from build123d import *

# Parameters (mm, degrees)
SKETCH1_W               = 94
SKETCH1_H               = 57
BOSS_EXTRUDE1_DEPTH     = 10
BOSS_EXTRUDE2_DEPTH     = 30
SKETCH3_W               = 1.5
SKETCH3_H               = 1.4
SKETCH3_W_2             = 1
SKETCH3_H_2             = 1
BOSS_EXTRUDE3_DEPTH     = 92
SKETCH3_3_W             = 1
SKETCH3_3_H             = 1
BOSS_EXTRUDE4_DEPTH     = 10
SKETCH4_W               = 46
SKETCH4_H               = 11
CUT_EXTRUDE1_DEPTH      = 10
SKETCH5_W               = 2
SKETCH5_H               = 2
CUT_EXTRUDE2_DEPTH      = 2
BOSS_EXTRUDE5_DEPTH     = 2
FILLET1_SIZE            = 1.5
BOSS_EXTRUDE6_DEPTH     = 1
SKETCH9_W               = 10
SKETCH9_H               = 2
BOSS_EXTRUDE7_DEPTH     = 2
CUT_EXTRUDE3_DEPTH      = 79.407264077
CUT_EXTRUDE3_DEPTH_BACK = 79.407264077
SKETCH10_W              = 52
SKETCH10_H              = 34
SKETCH11_W              = 92
SKETCH11_H              = 50
CUT_EXTRUDE4_DEPTH      = 2.2


with BuildPart() as part:
    # Sketch1 → Boss-Extrude1 (new body)
    with BuildSketch(Plane(origin=(0, 0, 0), x_dir=(1, 0, 0), z_dir=(0, 1, 0))):
        with Locations((16.701972288, 4.145945946)):
            Rectangle(SKETCH1_W, SKETCH1_H)
    extrude(amount=BOSS_EXTRUDE1_DEPTH)

    # Sketch2 → Boss-Extrude2 (add)
    with BuildSketch(Plane(origin=(0, 10, 0), x_dir=(1, 0, 0), z_dir=(0, 1, 0))):
        Polygon((-30.298027712, 32.645945946), (63.701972288, 32.645945946), (63.701972288, -24.354054054), (-30.298027712, -24.354054054), (-30.298027712, -22.354054054), (61.701972288, -22.354054054), (61.701972288, 30.645945946), (-30.298027712, 30.645945946), align=None)
    extrude(amount=BOSS_EXTRUDE2_DEPTH)

    # Sketch3 → Boss-Extrude3 (add)
    with BuildSketch(Plane.ZY.offset(30.298027712)):
        with Locations((-29.895945946, 10.7)):
            Rectangle(SKETCH3_W, SKETCH3_H)
        with Locations((21.604054054, 10.7)):
            Rectangle(SKETCH3_W, SKETCH3_H)
        with Locations((21.854054054, 14)):
            Rectangle(SKETCH3_W_2, SKETCH3_H_2)
    extrude(amount=-BOSS_EXTRUDE3_DEPTH)

    # Sketch3<3> → Boss-Extrude4 (add)
    with BuildSketch(Plane.ZY.offset(30.298027712)):
        with Locations((-30.145945946, 14)):
            Rectangle(SKETCH3_3_W, SKETCH3_3_H)
    extrude(amount=-BOSS_EXTRUDE4_DEPTH)

    # Sketch4 → Cut-Extrude1 (cut)
    with BuildSketch(Plane(origin=(0, 0, -32.645945946), x_dir=(-1, 0, 0), z_dir=(0, 0, -1))):
        with Locations((-33.701972288, 29)):
            Rectangle(SKETCH4_W, SKETCH4_H)
    extrude(amount=-CUT_EXTRUDE1_DEPTH, mode=Mode.SUBTRACT)

    # Sketch5 → Cut-Extrude2 (cut)
    with BuildSketch(Plane(origin=(63.701972288, 0, 0), x_dir=(0, 0, -1), z_dir=(1, 0, 0))):
        Polygon((-2.854054054, 30), (11.145945946, 30), (13.145945946, 28), (13.145945946, 14), (-4.854054054, 14), (-4.854054054, 28), align=None)
        with Locations((-7.854054054, 21)):
            Rectangle(SKETCH5_W, SKETCH5_H)
        with Locations((16.145945946, 21)):
            Rectangle(SKETCH5_W, SKETCH5_H)
    extrude(amount=-CUT_EXTRUDE2_DEPTH, mode=Mode.SUBTRACT)

    # Sketch7 → Boss-Extrude5 (add)
    with BuildSketch(Plane(origin=(0, 33, 0), x_dir=(1, 0, 0), z_dir=(0, 1, 0))):
        Polygon((10.701972288, -22.354054054), (61.701972288, -22.354054054), (61.701972288, -20.354054054), (61.701972288, 15.645945946), (59.701972288, 15.645945946), (59.701972288, -20.354054054), (10.701972288, -20.354054054), align=None)
    extrude(amount=-BOSS_EXTRUDE5_DEPTH)

    # Fillet1
    # a fillet whose section is not a circle: 1.5 mm, written as the material it takes off along each edge
    with BuildSketch(Plane(origin=(59.701972288, 31, -19.395945946), x_dir=(1, 0, 0), z_dir=(0, 0, 1))) as fillet1_piece_1:
        with BuildLine():
            Bezier((FILLET1_SIZE, 0), (0, 0), (0, FILLET1_SIZE), weights=[1, 0.353553391, 1])
            Line((0, FILLET1_SIZE), (0, 0))
            Line((0, 0), (FILLET1_SIZE, 0))
        make_face()
    extrude(amount=39.75, mode=Mode.SUBTRACT)
    with BuildSketch(Plane(origin=(59.701972288, 31, 20.354054054), x_dir=(0, 0, 1), z_dir=(-1, 0, 0))) as fillet1_piece_2:
        with BuildLine():
            Bezier((FILLET1_SIZE, 0), (0, 0), (0, FILLET1_SIZE), weights=[1, 0.353553391, 1])
            Line((0, FILLET1_SIZE), (0, 0))
            Line((0, 0), (FILLET1_SIZE, 0))
        make_face()
    extrude(amount=52.75, mode=Mode.SUBTRACT)
    with BuildSketch(Plane(origin=(59.701972288, 31, -19.395945946), x_dir=(1, 0, 0), z_dir=(0, 0, 1))) as fillet1_piece_3a_section:
        with BuildLine():
            Bezier((FILLET1_SIZE, 0), (0, 0), (0, FILLET1_SIZE), weights=[1, 0.353553391, 1])
            Line((0, FILLET1_SIZE), (0, 0))
            Line((0, 0), (FILLET1_SIZE, 0))
        make_face()
    fillet1_piece_3a = extrude(amount=43.5, mode=Mode.PRIVATE)
    fillet1_piece_3a = split(fillet1_piece_3a, bisect_by=Plane(origin=(59.701972288, 31, 22.354054054), z_dir=(0, 0, -1)), keep=Keep.TOP, mode=Mode.PRIVATE)
    fillet1_piece_3a = split(fillet1_piece_3a, bisect_by=Plane(origin=(59.701972288, 31, 20.354054054), z_dir=(0, 0, 1)), keep=Keep.TOP, mode=Mode.PRIVATE)
    with BuildSketch(Plane(origin=(63.451972288, 31, 20.354054054), x_dir=(0, 0, 1), z_dir=(-1, 0, 0))) as fillet1_piece_3b_section:
        with BuildLine():
            Bezier((FILLET1_SIZE, 0), (0, 0), (0, FILLET1_SIZE), weights=[1, 0.353553391, 1])
            Line((0, FILLET1_SIZE), (0, 0))
            Line((0, 0), (FILLET1_SIZE, 0))
        make_face()
    fillet1_piece_3b = extrude(amount=56.5, mode=Mode.PRIVATE)
    fillet1_piece_3b = split(fillet1_piece_3b, bisect_by=Plane(origin=(61.701972288, 31, 20.354054054), z_dir=(-1, 0, 0)), keep=Keep.TOP, mode=Mode.PRIVATE)
    fillet1_piece_3b = split(fillet1_piece_3b, bisect_by=Plane(origin=(59.701972288, 31, 20.354054054), z_dir=(1, 0, 0)), keep=Keep.TOP, mode=Mode.PRIVATE)
    fillet1_piece_3 = fillet1_piece_3a & fillet1_piece_3b
    add(fillet1_piece_3, mode=Mode.SUBTRACT)

    # Sketch8 → Boss-Extrude6 (add)
    with BuildSketch(Plane(origin=(0, 34.8, 0), x_dir=(1, 0, 0), z_dir=(0, 1, 0))):
        Polygon((10.701972288, -20.354054054), (59.701972288, -20.354054054), (59.701972288, 15.645945946), (61.701972288, 15.645945946), (61.701972288, -22.354054054), (10.701972288, -22.354054054), align=None)
    extrude(amount=BOSS_EXTRUDE6_DEPTH)

    # Sketch9 → Boss-Extrude7 (add)
    with BuildSketch(Plane(origin=(0, 40, 0), x_dir=(1, 0, 0), z_dir=(0, 1, 0))):
        with Locations((-25.298027712, 31.645945946)):
            Rectangle(SKETCH9_W, SKETCH9_H)
        with Locations((2.701972288, 31.645945946)):
            Rectangle(SKETCH9_W, SKETCH9_H)
        with Locations((30.701972288, 31.645945946)):
            Rectangle(SKETCH9_W, SKETCH9_H)
        with Locations((58.701972288, 31.645945946)):
            Rectangle(SKETCH9_W, SKETCH9_H)
        with Locations((-25.298027712, -23.354054054)):
            Rectangle(SKETCH9_W, SKETCH9_H)
        with Locations((2.701972288, -23.354054054)):
            Rectangle(SKETCH9_W, SKETCH9_H)
        with Locations((30.701972288, -23.354054054)):
            Rectangle(SKETCH9_W, SKETCH9_H)
        with Locations((58.701972288, -23.354054054)):
            Rectangle(SKETCH9_W, SKETCH9_H)
    extrude(amount=BOSS_EXTRUDE7_DEPTH)

    # Sketch10 → Cut-Extrude3 (cut, two sides: drawn at the far end of the back side and taken through both)
    with BuildSketch(Plane(origin=(0, 10, 0), x_dir=(1, 0, 0), z_dir=(0, 1, 0)).offset(-CUT_EXTRUDE3_DEPTH_BACK)):
        with Locations((5.701972288, 4.145945946)):
            Rectangle(SKETCH10_W, SKETCH10_H)
    extrude(amount=CUT_EXTRUDE3_DEPTH + CUT_EXTRUDE3_DEPTH_BACK, mode=Mode.SUBTRACT)

    # Sketch11 → Cut-Extrude4 (cut)
    with BuildSketch(Plane(origin=(0, 10, 0), x_dir=(1, 0, 0), z_dir=(0, 1, 0))):
        with Locations((15.701972288, 4.145945946)):
            Rectangle(SKETCH11_W, SKETCH11_H)
    extrude(amount=-CUT_EXTRUDE4_DEPTH, mode=Mode.SUBTRACT)


solid = part.part
Build history of the part. All positions in model axes, mm. A direction names the side the tool comes from. Give positions to 0.01 mm unless a question says otherwise; leave off trailing zeros. Loops run counter-clockwise (first coordinate to the right, second up) from the corner with the lowest first, then second, coordinate; pieces in that order, holes last. Notation, with made-up numbers: (45, 86.25) - (56, 86.25) arc R22 cw to (56, 116.25) - close; hole circle Ø6 at (26.5, 11.25). An arc over 180 degrees is marked (long way). Write item = value, one per line. Start each with the question number.
1) Drop flat-ended pins along their axis: pin 1 Ø1 at (x, z) = (-10.5, -32) entering from +Y; pin 2 Ø8 at (y, z) = (13, -6.5) entering from -X; pin 3 Ø6 at (x, z) = (-17, 7) entering from -Y; pin 4 Ø1 at (y, z) = (32, 21.5) entering from -X. Give the stop position or say it passes through.
2) Probe probe 1 along Y at (x, z) = (60.5, 8); probe 2 along Z at (x, y) = (19, 15); probe 3 along X at (y, z) = (37.5, -3). List the from-to ranges inside material, lowest first. Write a range as from..to.
3) Band-saw the part on C-C on y = 37. Give the cut face in (x, z), plus the area to 3 significant figures.
4) Tool access for faces 1 (the flat face through (45, 40, 23)), 2 (the flat face through (15, 12, 22.354)), 3 (the flat face through (62.716, 28.986, 3.868)), 4 (the flat face through (34, 23.5, -32)): list every direction of +Z, -Z, +X, -X, +Y, -Y with a clear straight run to the whole face (end or side of a thin tool).
5) Band-saw the part on A-A on y = 4. Give the cut face in (x, z), plus the area to 3 significant figures.
6) Band-saw the part on D-D on z = -8. Count the separate pieces of the cut face and the enclosed holes in it, plus the area to 3 significant figures.
7) Band-saw the part on B-B on x = -19. Give the cut face in (y, z), plus the area to 3 significant figures.
8) Pull direction Y, two halves, no side cores. Call faces 5 (the flat face through (7.702, 41, 23)), 6 (the flat face through (63, 21, 6.854)), 7 (the flat face through (-25, 42, -32)): +Y half, -Y half, draft (parallel to the pull), parting line (faces both ways), or undercut.
Final values:
q1.pin_1 = 40
q1.pin_2 = 61.7
q1.pin_3 = through
q1.pin_4 = 10.7
q2.probe_1 = 0..7.8, 31.34..33, 34.8..35.8
q2.probe_2 = -32.65..-30.65, 22.35..24.35
q2.probe_3 = 61.7..63.7
q3.outline = (-30.3, -32.65) - (63.7, -32.65) - (63.7, 24.35) - (-30.3, 24.35) - (-30.3, 22.35) - (61.7, 22.35) - (61.7, -30.65) - (-30.3, -30.65) - close
q3.area = 482 mm²
q4.face_1 = +Z, -Z, +Y
q4.face_2 = -X
q4.face_3 = +X, -X
q4.face_4 = -Z
q5.outline = (-30.3, -32.65) - (63.7, -32.65) - (63.7, 24.35) - (-30.3, 24.35) - close; hole (-20.3, -21.15) - (31.7, -21.15) - (31.7, 12.85) - (-20.3, 12.85) - close
q5.area = 3,590 mm²
q6.separate_pieces = 3
q6.enclosed_holes = 0
q6.area = 365 mm²
q7.outline = (0, -32.65) - (40, -32.65) - (40, -30.65) - (11.4, -30.65) - (11.4, -29.15) - (7.8, -29.15) - (7.8, -21.15) - (0, -21.15) - close; (0, 12.85) - (7.8, 12.85) - (7.8, 20.85) - (11.4, 20.85) - (11.4, 22.35) - (13.5, 22.35) - (13.5, 21.35) - (14.5, 21.35) - (14.5, 22.35) - (40, 22.35) - (40, 24.35) - (0, 24.35) - close
q7.area = 320 mm²
q8.face_5 = draft
q8.face_6 = undercut
q8.face_7 = +Y half
